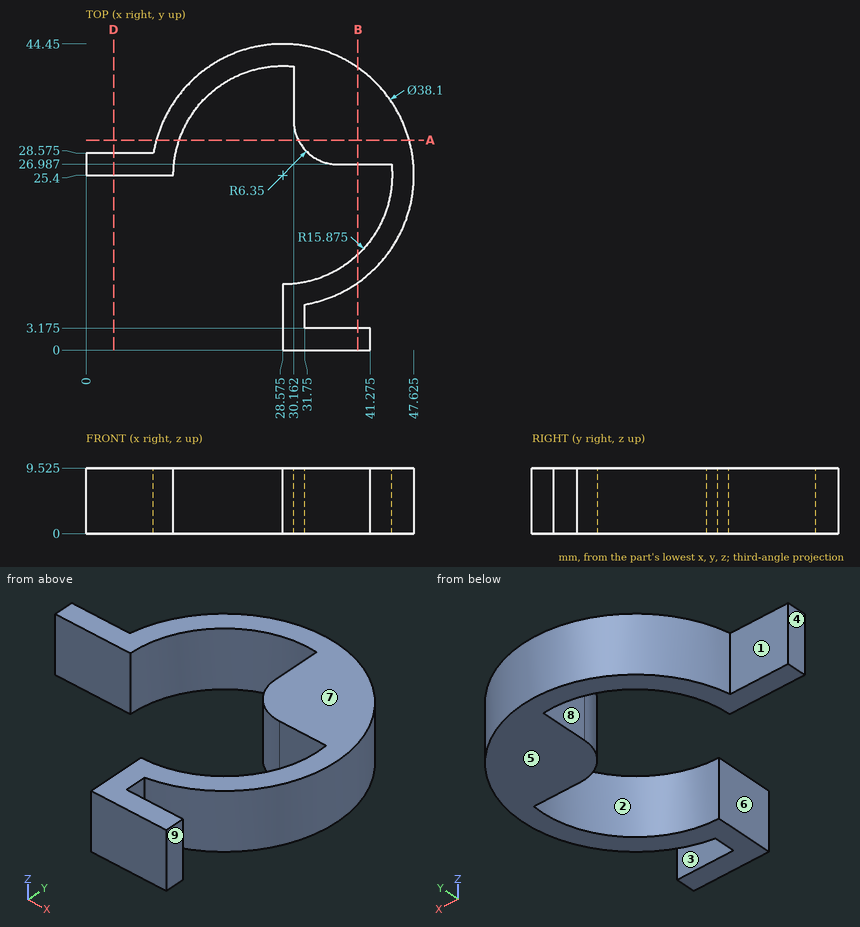
Could you check a few things on this drawing? It's one solid part, dimensions in mm from its lowest x, y, z. A direction names the side the tool comes from. Round coordinates to 2 decimals unless told otherwise and drop trailing zeros. Write each loop counter-clockwise with the first axis right and the second up, starting at its lowest first coordinate (ties: lowest second). Pieces come first, ordered by that corner, then holes. Notation, with made-up numbers: M 50,27.5 L 67,27.5 A31 cw 67,64.5 Z; hole C 60.25,29.5 d6. An arc over 180 degrees is marked long. Answer as CSV lines item,"result". Start each with the question number.
1. Suppose I cut it at B-B on x = 39.5. Write out the boundary of the cut face in (y, z) (1 decimal), then the cut area to 3 significant figures.
2. I need wall thicknesses on probe 1 along Y at (x, z) = (29, 5.75) (1 decimal); probe 2 along Y at (x, z) = (40, 5.25) (1 decimal); probe 3 along X at (y, z) = (35.5, 2) (1 decimal). Which ranges of each line are inside material? Lowest first, please.
3. Suppose I cut it at A-A on y = 30.5. Write out the boundary of the cut face in (x, z) (1 decimal), then the cut area to 3 significant figures.
4. Suppose I cut it at D-D on x = 4. Write out the boundary of the cut face in (y, z) (1 decimal).
5. On a 3-axis mill with a long thin cutter (end or side, diameter ignored), from which of +Z, -Z, +X, -X, +Y, -Y can I reach the whole of each face in a straight line? I mean the marked faces 5, 6, 7, 8 and 9. Say none if no direction works.
6. Thinking about a two-plate mould opening in Y: for the marked faces 1, 2, 3 and 4, which applies, released by +Y, released by -Y, zero draft, split by the parting line, or undercut?
7. I'm going to push flat-ended pins straight in: pin 1 Ø1.6 at (y, z) = (1.5, 7) entering from +X (1 decimal); pin 2 Ø5 at (x, z) = (5.5, 6.5) entering from +Y (1 decimal); pin 3 Ø5 at (y, z) = (13.5, 6) entering from -X (1 decimal); pin 4 Ø10 at (x, y) = (12, 37.5) entering from -Z. Where does each tip first touch, or does it pass through?
Check result:
1,outline,"M 0,0 L 3.2,0 L 3.2,9.5 L 0,9.5 Z; M 9.8,0 L 13.9,0 L 13.9,9.5 L 9.8,9.5 Z; M 27,0 L 41,0 L 41,9.5 L 27,9.5 Z"
1,area,"203 mm2"
2,probe 1,"y = 0 to 9.5, 41.3 to 44.4"
2,probe 2,"y = 0 to 3.2, 10.2 to 14.4, 27 to 40.6"
2,probe 3,"x = 12.4 to 16.3, 30.2 to 44.7"
3,outline,"M 10.2,0 L 13.5,0 L 13.5,9.5 L 10.2,9.5 Z; M 30.8,0 L 46.9,0 L 46.9,9.5 L 30.8,9.5 Z"
3,area,"185 mm2"
4,outline,"M 25.4,0 L 28.6,0 L 28.6,9.5 L 25.4,9.5 Z"
5,face 5,"-Z, +X, -X, +Y, -Y"
5,face 6,"+Z, -Z, -X, -Y"
5,face 7,"+Z, +X, -X, +Y, -Y"
5,face 8,"+Z, -Z"
5,face 9,"+Z, -Z, +X, -Y"
6,face 1,"released by +Y"
6,face 2,"undercut"
6,face 3,"undercut"
6,face 4,"zero draft"
7,pin 1,"stops at x = 41.3"
7,pin 2,"stops at y = 28.6"
7,pin 3,"stops at x = 35.3"
7,pin 4,"stops at z = 0"
